```python
from build123d import *

# Parameters (mm, degrees)
F0_W     = 50.8
F0_H     = 76.200003
F1_DEPTH = 38.1
F2_T     = -2.54
F3_W     = 45.72
F3_H     = 2.990683
F3_H_2   = 2.366999
F4_DEPTH = 35.56


with BuildPart() as f1:
    # F0 (on Top) → F1 (new body)
    with BuildSketch(Plane.XY):
        with Locations((4.165911, -5.146126)):
            Rectangle(F0_W, F0_H)
    extrude(amount=F1_DEPTH)

    # F2
    f2_openings = [f1.faces().sort_by_distance(p)[0] for p in [
        (4.165911, -5.146125, 38.1),
    ]]
    offset(amount=F2_T, openings=f2_openings)

    # F3 (on face) → F4 (join)
    with BuildSketch(Plane.XY.offset(2.54)):
        with Locations((4.165911, -3.650783)):
            Rectangle(F3_W, F3_H)
        with Locations((4.165911, -6.329624)):
            Rectangle(F3_W, F3_H_2)
    extrude(amount=F4_DEPTH)


solid = f1.part
```
Work out the finished part from the listing and answer in its coordinate system (mm). A direction names the side the tool comes from. Coordinates: 2 decimals unless noted, no trailing zeros. Order: outer loops, then holes, each group sorted by start corner. A loop starts at its lowest first (then second) coordinate and runs counter-clockwise, first axis right, second up. Notation, with made-up numbers: (-5, 88) - (30, 88) arc R26 cw to (30, 127) - close; hole circle Ø5 at (69.25, 7). An arc over 180 degrees is marked (long way). Answer as a JSON object with one key per item and string values.
1. Consider line 1 (Y direction, x = -17.5, z = 5.5); line 2 (X direction, y = 16, z = 6.5); line 3 (Z direction, x = -4.5, y = -28.5). Determine where each line is inside the solid, lowest interval first.
Output values:
{"line 1": "y = -43.25 to -40.71, -7.51 to -2.16, 30.41 to 32.95", "line 2": "x = -21.23 to -18.69, 27.03 to 29.57", "line 3": "z = 0 to 2.54"}
2. The mould has two halves that part along Y. Classify faces 1 (the face through (4, -43.246, 19)), 2 (the face through (-21.234, -6, 19)), 3 (the face through (4, -2.155, 20)): +Y half, -Y half, draft (parallel to the pull), parting line (faces both ways), or undercut.
Output values:
{"face 1": "-Y half", "face 2": "draft", "face 3": "undercut"}
3. This flat-tipped pin is pushed along its axis until it touches: P1, Ø16.5, axis at x = 2, y = 18.5, coming from the +Z side. Where does it stop, or does it pass through?
Output values:
{"P1": "stops at z = 2.54"}
4. A tool of negligible diameter and unlimited length cuts with its end or side. For faces 4 (the face through (4, 14, 2.54)), 5 (the face through (4, -5, 0)), from which of +Z, -Z, +X, -X, +Y, -Y can it reach the whole face along a straight path? Write none if from no direction.
Output values:
{"face 4": "+Z", "face 5": "-Z, +X, -X, +Y, -Y"}
5. Find section C-C on x = 23. Determine the outline of the cut face in (y, z), plus the area to 3 significant figures.
Output values:
{"outline": "(-43.25, 0) - (32.95, 0) - (32.95, 38.1) - (30.41, 38.1) - (30.41, 2.54) - (-2.16, 2.54) - (-2.16, 38.1) - (-7.51, 38.1) - (-7.51, 2.54) - (-40.71, 2.54) - (-40.71, 38.1) - (-43.25, 38.1) - close", "area": "565 mm²"}
6. Find section B-B on y = -9. Determine the outline of the cut face in (x, z), plus the area to 3 significant figures.
Output values:
{"outline": "(-21.23, 0) - (29.57, 0) - (29.57, 38.1) - (27.03, 38.1) - (27.03, 2.54) - (-18.69, 2.54) - (-18.69, 38.1) - (-21.23, 38.1) - close", "area": "310 mm²"}
7. Find section A-A on z = 13. Determine the outline of the cut face in (x, y), plus the area to 3 significant figures.
Output values:
{"outline": "(-21.23, -43.25) - (29.57, -43.25) - (29.57, 32.95) - (-21.23, 32.95) - close; hole (-18.69, -40.71) - (27.03, -40.71) - (27.03, -7.51) - (-18.69, -7.51) - close; hole (-18.69, -2.16) - (27.03, -2.16) - (27.03, 30.41) - (-18.69, 30.41) - close", "area": "864 mm²"}
